Geometry check sheet. Reference: the model listing, model coordinates, mm. A direction names the side the tool comes from. Coordinates: 2 decimals unless noted, no trailing zeros. Write each loop counter-clockwise with the first axis right and the second up, starting at its lowest first coordinate (ties: lowest second). Pieces come first, ordered by that corner, then holes. Notation, with made-up numbers: (13.5, 12) -> (23.5, 12) arc R17 cw to (23.5, 34) -> close; hole circle Ø5 at (0.25, 67). An arc over 180 degrees is marked (long way). Use a Markdown table: item, result.
```python
from build123d import *

# Parameters (mm, degrees)
CROQUIS1_W              = 70
CROQUIS1_H              = 60
CROQUIS1_R              = 12.5
SALIENTE_EXTRUIR1_DEPTH = 5
CROQUIS2_W              = 5.625
CROQUIS2_H              = 17
CROQUIS2_W_2            = 2.5
CROQUIS2_H_2            = 3.5
SALIENTE_EXTRUIR2_DEPTH = 32
CROQUIS3_R              = 5
SALIENTE_EXTRUIR3_DEPTH = 25
REDONDEO1_R             = 5


with BuildPart() as part:
    # Croquis1 → Saliente-Extruir1 (new body)
    with BuildSketch(Plane(origin=(0, 0, 0), x_dir=(1, 0, 0), z_dir=(0, 1, 0))):
        Rectangle(CROQUIS1_W, CROQUIS1_H)
        Circle(CROQUIS1_R, mode=Mode.SUBTRACT)
    extrude(amount=SALIENTE_EXTRUIR1_DEPTH)

    # Croquis2 → Saliente-Extruir2 (add)
    with BuildSketch(Plane.XZ):
        with Locations((32.1875, 0)):
            Rectangle(CROQUIS2_W, CROQUIS2_H)
        with Locations((28.125, 0)):
            Rectangle(CROQUIS2_W_2, CROQUIS2_H)
        with Locations((28.125, 10.25)):
            Rectangle(CROQUIS2_W_2, CROQUIS2_H_2)
        with Locations((24.0625, 0)):
            Rectangle(CROQUIS2_W, CROQUIS2_H)
        with Locations((28.125, -10.25)):
            Rectangle(CROQUIS2_W_2, CROQUIS2_H_2)
    extrude(amount=SALIENTE_EXTRUIR2_DEPTH)

    # Croquis3 → Saliente-Extruir3 (add)
    with BuildSketch(Plane(origin=(0, 5, 0), x_dir=(1, 0, 0), z_dir=(0, 1, 0))):
        with Locations((-25, 0)):
            Circle(CROQUIS3_R)
    extrude(amount=SALIENTE_EXTRUIR3_DEPTH)

    # Redondeo1
    redondeo1_edges = [part.edges().sort_by_distance(p)[0] for p in [
        (-30, 30, 0),
    ]]
    fillet(redondeo1_edges, radius=REDONDEO1_R)


solid = part.part
```
Item 1: Section check B-B on z = 0. Record the boundary of the cut face in (x, y), then the cut area to 3 significant figures.
Answer block:
| item | result |
|---|---|
| outline | (-35, 0) -> (-12.5, 0) -> (-12.5, 5) -> (-20, 5) -> (-20, 25) arc R5 ccw to (-30, 25) -> (-30, 5) -> (-35, 5) -> close; (12.5, 0) -> (21.25, 0) -> (21.25, -32) -> (35, -32) -> (35, 5) -> (12.5, 5) -> close |
| area | 904 mm^2 |
Item 2: Thickness scan on L1, parallel to X at y = 3, z = 0; L2, parallel to Z at x = 0, y = 1; L3, parallel to Y at x = 16.5, z = 5. Record the ranges inside material, lowest first. Write a range as [from, to].
Answer block:
| item | result |
|---|---|
| L1 | x = [-35, -12.5], [12.5, 35] |
| L2 | z = [-30, -12.5], [12.5, 30] |
| L3 | y = [0, 5] |
Item 3: Section check D-D on y = -25. Record the boundary of the cut face in (x, z) (3 decimals).
Answer block:
| item | result |
|---|---|
| outline | (21.25, -8.5) -> (26.875, -8.5) -> (26.875, -12) -> (29.375, -12) -> (29.375, -8.5) -> (35, -8.5) -> (35, 8.5) -> (29.375, 8.5) -> (29.375, 12) -> (26.875, 12) -> (26.875, 8.5) -> (21.25, 8.5) -> close |
Item 4: Depth check by flat-ended pin: P1, Ø3, axis at x = 28, y = -9.5, coming from the -Z side; P2, Ø3, axis at x = 25, y = -18, coming from the -Z side; P3, Ø1.2, axis at x = 28, y = -22, coming from the +Z side. Enter the tip coordinate at first touch or a pass-through.
Answer block:
| item | result |
|---|---|
| P1 | stops at z = -12 |
| P2 | stops at z = -8.5 |
| P3 | stops at z = 12 |
Item 5: Tool access check on faces 1 (the flat face through (26.875, -16, 10)), 2 (the flat face through (26.875, -16, -10)), 3 (the flat face through (28, -16, -12)). Record the directions out of +Z, -Z, +X, -X, +Y, -Y that give a thin tool (end or side, any length) a straight path to the whole face; none if there is none.
Answer block:
| item | result |
|---|---|
| face 1 | +Z, -X, -Y |
| face 2 | -Z, -X, -Y |
| face 3 | -Z, +X, -X, -Y |
Item 6: Section check A-A on x = 0. Record the boundary of the cut face in (y, z).
Answer block:
| item | result |
|---|---|
| outline | (0, -30) -> (5, -30) -> (5, -12.5) -> (0, -12.5) -> close; (0, 12.5) -> (5, 12.5) -> (5, 30) -> (0, 30) -> close |
Item 7: Section check C-C on x = 25.5. Record the boundary of the cut face in (y, z), then the cut area to 3 significant figures.
Answer block:
| item | result |
|---|---|
| outline | (-32, -8.5) -> (0, -8.5) -> (0, -30) -> (5, -30) -> (5, 30) -> (0, 30) -> (0, 8.5) -> (-32, 8.5) -> close |
| area | 844 mm^2 |
